Here's how the part is built. I have some questions about the finished solid (model axes, mm). A direction names the side the tool comes from. Coordinates: 2 decimals unless noted, no trailing zeros. Order: outer loops, then holes, each group sorted by start corner. A loop starts at its lowest first (then second) coordinate and runs counter-clockwise, first axis right, second up.
```python
from build123d import *

# Parameters (mm, degrees)
SKETCH_2_R                = 150
EXTRUDE_1_DEPTH           = 15
SKETCH_3_R                = 35
CUT_EXTRUDE_1_DEPTH       = 3
EXTRUDE_START             = 16.5
SKETCH_4_R                = 38.5
SKETCH_4_R_2              = 35
EXTRUDE_2_DEPTH           = 16.5
EXTRUDE_START_2           = 13.5
SKETCH_5_R                = 46.5
SKETCH_5_R_2              = 38.5
EXTRUDE_3_DEPTH           = 13.5
CHAMFER_1_SIZE            = 0.5
HOLE_WIZARD_1_D           = 6.6
HOLE_WIZARD_1_CBORE_D     = 11
HOLE_WIZARD_1_CBORE_DEPTH = 8
HOLE_WIZARD_6_0_6_1_D     = 6
CHAMFER_3_SIZE            = 1
CUT_EXTRUDE_START         = 69
SKETCH_20_R               = 46.5
CUT_EXTRUDE_5_DEPTH       = 69
SKETCH_22_R               = 4
CUT_EXTRUDE_7_DEPTH       = 244.812402925
CHAMFER_6_SIZE            = 1
HOLE_WIZARD_M8_1_D        = 6.8
EXTRUDE_START_3           = 5
SKETCH_27_R               = 40
SKETCH_27_R_2             = 35
EXTRUDE_4_DEPTH           = 5
CHAMFER_7_SIZE            = 0.5
CHAMFER_8_SIZE            = 2
SKETCH_25_R               = 20
CUT_EXTRUDE_8_DEPTH       = 245.171021663
CHAMFER_9_SIZE            = 2
FILLET_1_R                = 1
SKETCH_28_OUTSIDE_W       = 386.948
SKETCH_28_OUTSIDE_H       = 386.948
SKETCH_28_OUTSIDE_R       = 110
CUT_EXTRUDE_9_DEPTH       = 245.171021663
SKETCH_29_W               = 180
SKETCH_29_H               = 198.338891977
EXTRUDE_5_DEPTH           = 15


with BuildPart() as part:
    # 草图2 → 凸台-拉伸1 (new body)
    with BuildSketch(Plane.XY.offset(1)):
        with Locations((18.556612769, -25.522523089)):
            Circle(SKETCH_2_R)
    extrude(amount=EXTRUDE_1_DEPTH)

    # 草图3 → 切除-拉伸1 (cut)
    with BuildSketch(Plane(origin=(0, 0, 1), x_dir=(-1, 0, 0), z_dir=(0, 0, -1))):
        with Locations((-18.556612769, -25.522523089)):
            Circle(SKETCH_3_R)
    extrude(amount=-CUT_EXTRUDE_1_DEPTH, mode=Mode.SUBTRACT)

    # 草图4 → 凸台-拉伸2 (add)
    with BuildSketch(Plane(origin=(0, 0, 1), x_dir=(-1, 0, 0), z_dir=(0, 0, -1)).offset(EXTRUDE_START)):
        with Locations(Location((-18.556612769, -25.522523089, 0), (0, 0, 180))):
            Circle(SKETCH_4_R)
        with Locations((-18.556612769, -25.522523089)):
            Circle(SKETCH_4_R_2, mode=Mode.SUBTRACT)
    extrude(amount=-EXTRUDE_2_DEPTH)

    # 草图5 → 凸台-拉伸3 (add)
    with BuildSketch(Plane(origin=(0, 0, 1), x_dir=(-1, 0, 0), z_dir=(0, 0, -1)).offset(EXTRUDE_START_2)):
        with Locations(Location((-18.556612769, -25.522523089, 0), (0, 0, 180))):
            Circle(SKETCH_5_R)
        with Locations(Location((-18.556612769, -25.522523089, 0), (0, 0, 90))):
            Circle(SKETCH_5_R_2, mode=Mode.SUBTRACT)
    extrude(amount=-EXTRUDE_3_DEPTH)

    # 倒角1
    chamfer_1_edges = [part.edges().sort_by_distance(p)[0] for p in [
        (53.556612769, -25.522523089, -15.5),
        (-19.943387231, -25.522523089, -15.5),
    ]]
    chamfer(chamfer_1_edges, length=CHAMFER_1_SIZE)

    # 打孔尺寸根据内六角圆柱头螺钉的类型1 (through all)
    with Locations(Plane(origin=(42.626407432, -13.463363362, 16), x_dir=(1, 0, 0), z_dir=(0, 0, 1))):
        with Locations((-41.703352232, 12.211350104), (-6.436237094, 12.211350104), (4.461900826, -21.329669558), (-52.601490152, -21.329669558)):
            CounterBoreHole(HOLE_WIZARD_1_D / 2, HOLE_WIZARD_1_CBORE_D / 2, HOLE_WIZARD_1_CBORE_DEPTH)

    # Ø6.0 (6) 直径孔1 (through all)
    with Locations(Plane.XY.offset(16)):
        with Locations((18.556612769, -55.522523089)):
            Hole(HOLE_WIZARD_6_0_6_1_D / 2)

    # 倒角3
    chamfer_3_edges = [part.edges().sort_by_distance(p)[0] for p in [
        (21.556612769, -55.522523089, 16),
    ]]
    chamfer(chamfer_3_edges, length=CHAMFER_3_SIZE)

    # 草图20 → 切除-拉伸5 (cut)
    with BuildSketch(Plane(origin=(0, 0, 1), x_dir=(-1, 0, 0), z_dir=(0, 0, -1)).offset(CUT_EXTRUDE_START)):
        with Locations((-18.556612769, -25.522523089)):
            Circle(SKETCH_20_R)
    extrude(amount=-CUT_EXTRUDE_5_DEPTH, mode=Mode.SUBTRACT)

    # 草图22 → 切除-拉伸7 (cut, through all)
    with BuildSketch(Plane.XY.offset(16)):
        with Locations((-1.443387231, -68.522523089)):
            Circle(SKETCH_22_R)
        with Locations((38.556612769, -68.522523089)):
            Circle(SKETCH_22_R)
    extrude(amount=-CUT_EXTRUDE_7_DEPTH, mode=Mode.SUBTRACT)

    # 倒角6
    chamfer_6_edges = [part.edges().sort_by_distance(p)[0] for p in [
        (-5.443387231, -68.522523089, 16),
        (34.556612769, -68.522523089, 16),
    ]]
    chamfer(chamfer_6_edges, length=CHAMFER_6_SIZE)

    # M8 螺纹孔1 (through all)
    with Locations(Plane.XY.offset(16)):
        with Locations((-31.443387231, -43.522523089), (-31.443387231, -63.522523089), (68.556612769, -43.522523089), (68.556612769, -63.522523089), (18.556612769, -25.522523089)):
            Hole(HOLE_WIZARD_M8_1_D / 2)

    # 草图27 → 凸台-拉伸4 (add)
    with BuildSketch(Plane(origin=(0, 0, 1), x_dir=(-1, 0, 0), z_dir=(0, 0, -1)).offset(EXTRUDE_START_3)):
        with Locations(Location((-18.556612769, -25.522523089, 0), (0, 0, 180))):
            Circle(SKETCH_27_R)
        with Locations((-18.556612769, -25.522523089)):
            Circle(SKETCH_27_R_2, mode=Mode.SUBTRACT)
    extrude(amount=-EXTRUDE_4_DEPTH)

    # 倒角7
    chamfer_7_edges = [part.edges().sort_by_distance(p)[0] for p in [
        (53.556612769, -25.522523089, -4),
    ]]
    chamfer(chamfer_7_edges, length=CHAMFER_7_SIZE)

    # 倒角8
    chamfer_8_edges = [part.edges().sort_by_distance(p)[0] for p in [
        (-131.443387231, -25.522523089, 1),
        (-131.443387231, -25.522523089, 16),
    ]]
    chamfer(chamfer_8_edges, length=CHAMFER_8_SIZE)

    # 草图25 → 切除-拉伸8 (cut, through all)
    with BuildSketch(Plane.XY.offset(16)):
        with Locations((18.556612769, -25.522523089)):
            Circle(SKETCH_25_R)
    extrude(amount=-CUT_EXTRUDE_8_DEPTH, mode=Mode.SUBTRACT)

    # 倒角9
    chamfer_9_edges = [part.edges().sort_by_distance(p)[0] for p in [
        (-1.443387231, -25.522523089, 4),
        (-1.443387231, -25.522523089, 16),
    ]]
    chamfer(chamfer_9_edges, length=CHAMFER_9_SIZE)

    # 圆角1
    fillet_1_edges = [part.edges().sort_by_distance(p)[0] for p in [
        (-21.443387231, -25.522523089, 1),
    ]]
    fillet(fillet_1_edges, radius=FILLET_1_R)

    # 草图28 outside → 切除-拉伸9 (cut, through all)
    with BuildSketch(Plane.XY.offset(16)):
        with Locations((18.557, -25.523)):
            Rectangle(SKETCH_28_OUTSIDE_W, SKETCH_28_OUTSIDE_H)
        with Locations((18.556612769, -25.522523089)):
            Circle(SKETCH_28_OUTSIDE_R, mode=Mode.SUBTRACT)
    extrude(amount=-CUT_EXTRUDE_9_DEPTH, mode=Mode.SUBTRACT)

    # 草图29 → 凸台-拉伸5 (add)
    with BuildSketch(Plane.XY.offset(16)):
        with Locations((18.556612769, -181.353077101)):
            Rectangle(SKETCH_29_W, SKETCH_29_H)
    extrude(amount=-EXTRUDE_5_DEPTH)


solid = part.part
```
Q1. For faces 1 (the flat face through (-6, -35, 8)), 2 (the cylindrical face through (-1.964, -64.557, 8.098)), which set-ups out of +Z, -Z, +X, -X, +Y, -Y let a thin tool reach every point of the face, with its end or its side?
Q2. I need wall thicknesses on L1, parallel to X at y = -29, z = 14.25; L2, parallel to Y at x = 1.5, z = 7.25; L3, parallel to Y at x = 36.5, z = 5.25. Which ranges of each line are inside material? Lowest first, please.
Q3. We'd pull the mould along X, two halves only. Please class faces 3 (the flat face through (-71.443, -186, 9)), 4 (the flat face through (17, -95, 16)), 5 (the flat face through (35, -41, 4)): pulls with the +X half, pulls with the -X half, needs draft (parallel to the pull), parting line crosses it, or undercut.
Q4. Will these pins go through, and if not, where does the flat tip stop? pin 1 (6 mm diameter, centred on x = -31.44, y = -63.52, fed in from +Z); pin 2 (8 mm diameter, centred on y = -215.5, z = 10, fed in from +X); pin 3 (4 mm diameter, centred on y = -162.5, z = 13.5, fed in from -X); pin 4 (21 mm diameter, centred on x = 17.5, y = -42.5, fed in from -Z).
Q5. If we section it at A-A on y = -168: Write out the boundary of the cut face in (x, z), then the cut area to 3 significant figures.
Q6. If we section it at B-B on x = 104: Write out the boundary of the cut face in (y, z).
Reply:
1. face 1: +Z
1. face 2: +Z, -Z
2. L1: x = -91.39 to -1.39, 38.51 to 128.5
2. L2: y = -280.52 to -71.23, -65.81 to -35.97, -15.08 to -4.5, 2 to 83.15
2. L3: y = -280.52 to -71.95, -65.09 to -35.94, -15.1 to -4.54, 2.03 to 83
3. face 3: pulls with the -X half
3. face 4: needs draft
3. face 5: undercut
4. pin 1: passes through
4. pin 2: stops at x = 108.56
4. pin 3: stops at x = -71.44
4. pin 4: stops at z = 4
5. outline: (-71.44, 1) - (108.56, 1) - (108.56, 16) - (-71.44, 16) - close
5. area: 2,700 mm2
6. outline: (-280.52, 1) - (43.76, 1) - (43.76, 16) - (-280.52, 16) - close
